Work out the finished part from the listing and answer in its coordinate system (mm). A direction names the side the tool comes from. Give positions to 0.01 mm unless a question says otherwise; leave off trailing zeros. Order: outer loops, then holes, each group sorted by start corner. A loop starts at its lowest first (then second) coordinate and runs counter-clockwise, first axis right, second up.
```python
from build123d import *

# Parameters (mm, degrees)
SKETCH1_W                    = 25.4
SKETCH1_H                    = 101.6
BASE_FLANGE1_DEPTH           = 3.175
EDGE_FLANGE1_STRIP_W         = 18.7
EDGE_FLANGE1_STRIP_H         = 3.175
EDGE_FLANGE1_STRIP_CUT_DEPTH = 101.6
EDGE_FLANGE1_DEPTH           = 101.6
EDGE_FLANGE2_STRIP_W         = 18.7
EDGE_FLANGE2_STRIP_H         = 3.175
EDGE_FLANGE2_STRIP_CUT_DEPTH = 101.6
EDGE_FLANGE2_DEPTH           = 101.6
F_11_0_191_DIAMETER_HOLE1_D  = 4.8514
FILLET1_R                    = 6.35


# Sheet-metal steps are written as plain solids
with BuildPart() as part:
    # Sketch1 → Base-Flange1 (new body)
    with BuildSketch(Plane.XY):
        with Locations((-12.7, -50.8)):
            Rectangle(SKETCH1_W, SKETCH1_H)
    extrude(amount=-BASE_FLANGE1_DEPTH)

    # Edge-Flange1 strip (across the edge) → Edge-Flange1 strip cut (cut)
    with BuildSketch(Plane(origin=(-25.4, -101.6, -3.175), x_dir=(1, 0, 0), z_dir=(0, 1, 0))):
        with Locations((-3.175, -1.5875)):
            Rectangle(EDGE_FLANGE1_STRIP_W, EDGE_FLANGE1_STRIP_H)
    extrude(amount=EDGE_FLANGE1_STRIP_CUT_DEPTH, mode=Mode.SUBTRACT)

    # Edge-Flange1 section (across the edge) → Edge-Flange1 (add)
    with BuildSketch(Plane(origin=(-25.4, -101.6, -3.175), x_dir=(1, 0, 0), z_dir=(0, 1, 0))):
        with BuildLine():
            Line((0, 3), (0, 19.05))
            Line((0, 19.05), (3.175, 19.05))
            Line((3.175, 19.05), (3.175, 3))
            ThreePointArc((3.175, 3), (4.053679656, 0.878679656), (6.175, 0))
            Line((6.175, 0), (6.175, -3.175))
            ThreePointArc((6.175, -3.175), (1.808615626, -1.366384374), (0, 3))
        make_face()
    extrude(amount=EDGE_FLANGE1_DEPTH)

    # Edge-Flange2 strip (across the edge) → Edge-Flange2 strip cut (cut)
    with BuildSketch(Plane(origin=(-25.4, 0, -22.225), x_dir=(0, 0, 1), z_dir=(0, -1, 0))):
        with Locations((-6.35, -1.5875)):
            Rectangle(EDGE_FLANGE2_STRIP_W, EDGE_FLANGE2_STRIP_H)
    extrude(amount=EDGE_FLANGE2_STRIP_CUT_DEPTH, mode=Mode.SUBTRACT)

    # Edge-Flange2 section (across the edge) → Edge-Flange2 (add)
    with BuildSketch(Plane(origin=(-25.4, 0, -22.225), x_dir=(0, 0, 1), z_dir=(0, -1, 0))):
        with BuildLine():
            Line((-3.175, 3), (-3.175, 28.575))
            Line((-3.175, 28.575), (0, 28.575))
            Line((0, 28.575), (0, 3))
            ThreePointArc((0, 3), (0.878679656, 0.878679656), (3, 0))
            Line((3, 0), (3, -3.175))
            ThreePointArc((3, -3.175), (-1.366384374, -1.366384374), (-3.175, 3))
        make_face()
    extrude(amount=EDGE_FLANGE2_DEPTH)

    # #11 (0.191) Diameter Hole1 (through all)
    with Locations(Plane.XY):
        with Locations((-6.35, -12.7), (-6.35, -88.9)):
            Hole(F_11_0_191_DIAMETER_HOLE1_D / 2)

    # Fillet1
    fillet1_edges = [part.edges().sort_by_distance(p)[0] for p in [
        (-53.975, 0, -23.8125),
        (-53.975, -101.6, -23.8125),
        (0, -101.6, -1.5875),
        (0, 0, -1.5875),
    ]]
    fillet(fillet1_edges, radius=FILLET1_R)


solid = part.part
```
1. The part is cut by section A-A (y = -88.9). Write down the section's boundary in (x, z) (3 decimals).
Findings below:
outline: (-53.975, -25.4) - (-28.4, -25.4) arc R6.175 ccw to (-22.225, -19.225) - (-22.225, -6.175) arc R3 cw to (-19.225, -3.175) - (-8.776, -3.175) - (-8.776, 0) - (-19.225, 0) arc R6.175 ccw to (-25.4, -6.175) - (-25.4, -19.225) arc R3 cw to (-28.4, -22.225) - (-53.975, -22.225) - close; (-3.924, -3.175) - (0, -3.175) - (0, 0) - (-3.924, 0) - close
2. Given P1, Ø4, axis at x = -29.5, z = -20, coming from the -Y side; P2, Ø4, axis at x = -11.5, y = -31.5, coming from the -Z side (3 decimals); P3, Ø3, axis at x = -22.5, y = -44, coming from the +Z side; P4, Ø8, axis at y = -54.5, z = -18.5, coming from the +X side (3 decimals), each flat-ended and moving along its own axis, determine where each tip first touches the part or whether it passes through.
Findings below:
P1: passes through
P2: stops at z = -3.175
P3: stops at z = -0.26
P4: stops at x = -22.225
3. Straight lines are drawn through the part: probe 1 along Z at (x, y) = (-5.5, -9.5) (3 decimals); probe 2 along Y at (x, z) = (-7, -2); probe 3 along X at (y, z) = (-10, -16.5) (3 decimals). For each, find the intervals that lie inside material, in ascending order.
Findings below:
probe 1: z = -3.175 to 0
probe 2: y = -101.6 to -91.24, -86.56 to -15.04, -10.36 to 0
probe 3: x = -25.4 to -22.225
4. Which of the six approach directions +Z, -Z, +X, -X, +Y, -Y give full straight-line access (tool end or side, diameter ignored) to faces 1 (the face through (-10, -50, -3.175)), 2 (the face through (-25.4, -52, -13)), 3 (the face through (-1.91, -1.81, -1.61))?
Findings below:
face 1: -Z, +X, +Y, -Y
face 2: +Z, -X, +Y, -Y
face 3: +Z, -Z, +X, +Y
5. The part is cut by section C-C (x = -12.5). Write down the section's boundary in (y, z) (3 decimals), then the cut area to 3 significant figures.
Findings below:
outline: (-101.6, -3.175) - (0, -3.175) - (0, 0) - (-101.6, 0) - close
area: 323 mm2
6. The mould has two halves that part along Y. Classify faces 4 (the face through (-22.225, -52, -13)), 5 (the face through (-24, -101.6, -14)), 6 (the face through (-7.47, -91.05, -1.61)): pulls with the +Y half, pulls with the -Y half, needs draft (parallel to the pull), parting line crosses it, or undercut.
Findings below:
face 4: needs draft
face 5: pulls with the -Y half
face 6: undercut
7. The part is cut by section B-B (y = -77). Write down the section's boundary in (x, z) (3 decimals).
Findings below:
outline: (-53.975, -25.4) - (-28.4, -25.4) arc R6.175 ccw to (-22.225, -19.225) - (-22.225, -6.175) arc R3 cw to (-19.225, -3.175) - (0, -3.175) - (0, 0) - (-19.225, 0) arc R6.175 ccw to (-25.4, -6.175) - (-25.4, -19.225) arc R3 cw to (-28.4, -22.225) - (-53.975, -22.225) - close
